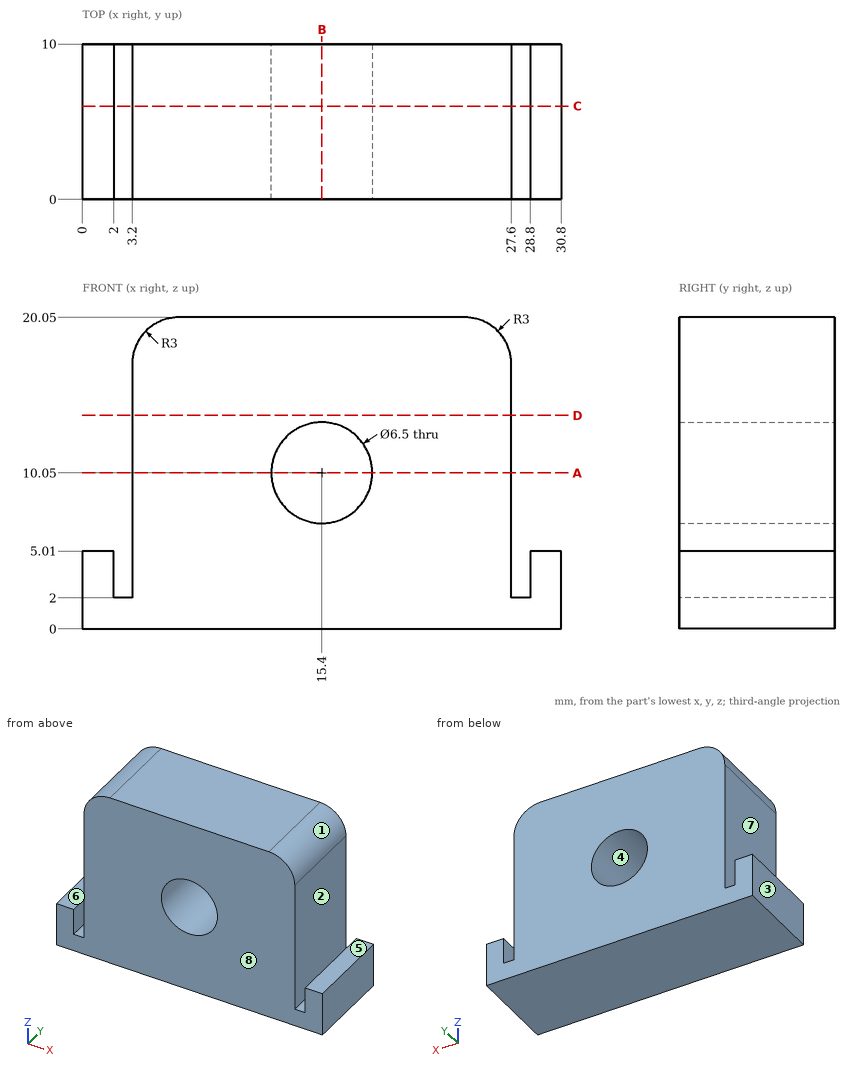
Print and shaded views of the part. All mm, measured from the part's lowest x, y and z. A direction names the side the tool comes from. Give positions to 0.01 mm unless a question says otherwise; leave off trailing zeros. Loops run counter-clockwise (first coordinate to the right, second up) from the corner with the lowest first, then second, coordinate; pieces in that order, holes last. Notation, with made-up numbers: (11, 40.25) -> (66, 40.25) arc R23 ccw to (66, 55.25) -> close; hole circle Ø8 at (-5, 40.5). An arc over 180 degrees is marked (long way). Use CSV: the item, a comma, the result in double quotes. Start each with the question number.
1) Slice it at C-C on y = 6. Give the cut face in (x, z).
2) Slice it at B-B on x = 15.4. Give the cut face in (y, z).
3) Tool access for the marked faces 4, 5, 6, 7 and 8: list every direction of +Z, -Z, +X, -X, +Y, -Y with a clear straight run to the whole face (end or side of a thin tool).
4) Wall check: line 1 (X direction, y = 9.25, z = 4.5); line 2 (Z direction, x = 15.4, y = 3.75); line 3 (Z direction, x = 18, y = 4.75). Give the ranges that are in metal, low to high.
5) Mould opens along X. For the marked faces 1, 2 and 3 say: released by +X, released by -X, zero draft, split by the parting line, or undercut.
6) Flat gauge pins, fed straight in: pin 1 Ø5 at (y, z) = (5.5, 10) entering from +X; pin 2 Ø0.6 at (x, y) = (2.5, 3) entering from +Z; pin 3 Ø3 at (y, z) = (6.5, 12) entering from -X. Where does each tip first touch, or does it go through?
7) Slice it at D-D on z = 13.75. Give the cut face in (x, y), plus the area to 3 significant figures.
8) Slice it at A-A on z = 10.05. Give the cut face in (x, y).
Computed values:
1,outline,"(0, 0) -> (30.8, 0) -> (30.8, 5.01) -> (28.8, 5.01) -> (28.8, 2) -> (27.6, 2) -> (27.6, 17.05) arc R3 ccw to (24.6, 20.05) -> (6.2, 20.05) arc R3 ccw to (3.2, 17.05) -> (3.2, 2) -> (2, 2) -> (2, 5.01) -> (0, 5.01) -> close; hole circle Ø6.5 at (15.4, 10.05)"
2,outline,"(0, 0) -> (10, 0) -> (10, 6.8) -> (0, 6.8) -> close; (0, 13.3) -> (10, 13.3) -> (10, 20.05) -> (0, 20.05) -> close"
3,face 4,"+Y, -Y"
3,face 5,"+Z, +X, +Y, -Y"
3,face 6,"+Z, -X, +Y, -Y"
3,face 7,"+Z, +Y, -Y"
3,face 8,"+Z, -Z, +X, -X, -Y"
4,line 1,"x = 0 to 2, 3.2 to 27.6, 28.8 to 30.8"
4,line 2,"z = 0 to 6.8, 13.3 to 20.05"
4,line 3,"z = 0 to 8.1, 12 to 20.05"
5,face 1,"released by +X"
5,face 2,"undercut"
5,face 3,"released by -X"
6,pin 1,"stops at x = 27.6"
6,pin 2,"stops at z = 2"
6,pin 3,"stops at x = 3.2"
7,outline,"(3.2, 0) -> (27.6, 0) -> (27.6, 10) -> (3.2, 10) -> close"
7,area,"244 mm^2"
8,outline,"(3.2, 0) -> (12.15, 0) -> (12.15, 10) -> (3.2, 10) -> close; (18.65, 0) -> (27.6, 0) -> (27.6, 10) -> (18.65, 10) -> close"
